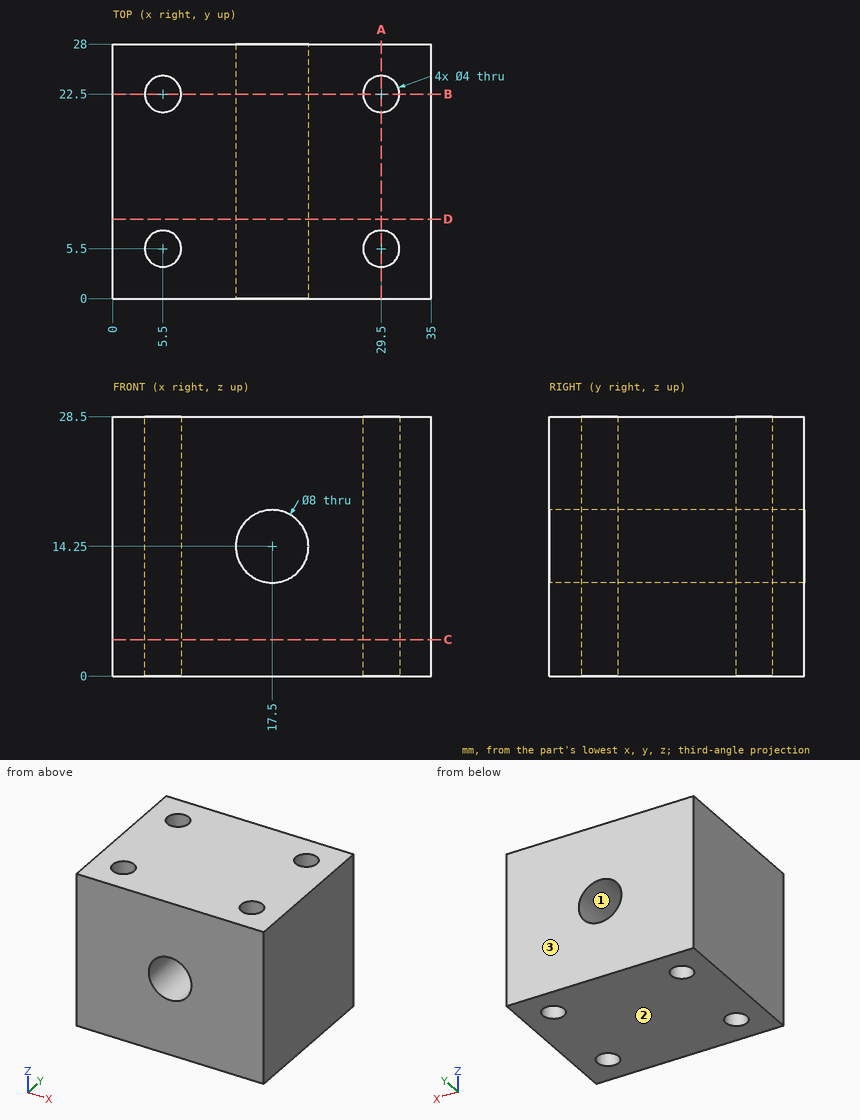
Geometry: see drawing. Coordinates: mm, zero at the bounding-box minimum. Give positions to 0.01 mm unless a question says otherwise; leave off trailing zeros. Order: outer loops, then holes, each group sorted by start corner. A loop starts at its lowest first (then second) coordinate and runs counter-clockwise, first axis right, second up. Notation, with made-up numbers: (-30, 22.25) - (-7, 22.25) arc R30 ccw to (-7, 46.25) - close; hole circle Ø10 at (1, 16). An arc over 180 degrees is marked (long way). One line per item, written item: value.
1. Draft query along Z for the marked faces 1, 2 and 3. Return one class per face: released by +Z, released by -Z, zero draft, split by the parting line, or undercut.
Determined:
face 1: undercut
face 2: released by -Z
face 3: zero draft
2. Cut plane A-A, the plane x = 29.5. Output: boundary loops of the cut face in (y, z), and give its area (3 significant figures).
Determined:
outline: (0, 0) - (3.5, 0) - (3.5, 28.5) - (0, 28.5) - close; (7.5, 0) - (20.5, 0) - (20.5, 28.5) - (7.5, 28.5) - close; (24.5, 0) - (28, 0) - (28, 28.5) - (24.5, 28.5) - close
area: 570 mm2
3. Pin query (flat end, axial travel): pin 1 Ø2.5 at (x, y) = (29.5, 5.5) entering from -Z. Return the tip coordinate at first contact, or that it passes through.
Determined:
pin 1: through
4. Cut plane D-D, the plane y = 8.75. Output: boundary loops of the cut face in (x, z).
Determined:
outline: (0, 0) - (35, 0) - (35, 28.5) - (0, 28.5) - close; hole circle Ø8 at (17.5, 14.25)
5. Cut plane B-B, the plane y = 22.5. Output: boundary loops of the cut face in (x, z).
Determined:
outline: (0, 0) - (3.5, 0) - (3.5, 28.5) - (0, 28.5) - close; (7.5, 0) - (27.5, 0) - (27.5, 28.5) - (7.5, 28.5) - close; (31.5, 0) - (35, 0) - (35, 28.5) - (31.5, 28.5) - close; hole circle Ø8 at (17.5, 14.25)
6. Cut plane C-C, the plane z = 4. Output: boundary loops of the cut face in (x, y), and give its area (3 significant figures).
Determined:
outline: (0, 0) - (35, 0) - (35, 28) - (0, 28) - close; hole circle Ø4 at (5.5, 5.5); hole circle Ø4 at (5.5, 22.5); hole circle Ø4 at (29.5, 5.5); hole circle Ø4 at (29.5, 22.5)
area: 930 mm2
7. Line query: probe 1 along Y at (x, z) = (29.5, 8); probe 2 along X at (y, z) = (22.5, 21.25); probe 3 along Y at (x, z) = (4, 10.25). Output: solid intervals per line, ascending.
Determined:
probe 1: 0 to 3.5, 7.5 to 20.5, 24.5 to 28
probe 2: 0 to 3.5, 7.5 to 27.5, 31.5 to 35
probe 3: 0 to 4.18, 6.82 to 21.18, 23.82 to 28
